from build123d import *

# Parameters (mm, degrees)
SKETCH3_W            = 36.5
SKETCH3_H            = 37.1
SHELL_DEPTH          = 8.6
SKETCH4_W            = 32.5
SKETCH4_H            = 31.1
MAIN_CAVITY_DEPTH    = 6.6
SKETCH5_W            = 32.5
SKETCH5_H            = 2
SUPPORT_SHELF_DEPTH  = 4.6
TERMINAL_INPUT_DEPTH = 2
SKETCH7_W            = 1.8
SKETCH7_H            = 3.6
MALE_TABS_DEPTH      = 2
SKETCH8_W            = 2
SKETCH8_H            = 4
FEMALE_TABS_DEPTH    = 2


with BuildPart() as part:
    # Sketch3 → Shell (new body)
    with BuildSketch(Plane(origin=(0, 0, 0), x_dir=(1, 0, 0), z_dir=(0, 1, 0))):
        with Locations((18.25, -18.55)):
            Rectangle(SKETCH3_W, SKETCH3_H)
    extrude(amount=SHELL_DEPTH)

    # Sketch4 → Main Cavity (cut)
    with BuildSketch(Plane(origin=(0, 8.6, 0), x_dir=(1, 0, 0), z_dir=(0, 1, 0))):
        with Locations((18.25, -19.55)):
            Rectangle(SKETCH4_W, SKETCH4_H)
    extrude(amount=-MAIN_CAVITY_DEPTH, mode=Mode.SUBTRACT)

    # Sketch5 → Support Shelf (cut)
    with BuildSketch(Plane(origin=(0, 8.6, 0), x_dir=(1, 0, 0), z_dir=(0, 1, 0))):
        with Locations((18.25, -3)):
            Rectangle(SKETCH5_W, SKETCH5_H)
    extrude(amount=-SUPPORT_SHELF_DEPTH, mode=Mode.SUBTRACT)

    # Sketch6 → Terminal Input (cut)
    with BuildSketch(Plane.XY.offset(37.1)):
        Polygon((31.2, 2.9), (31.2, 8.6), (4.1, 8.6), (4.1, 0), (14.7, 0), (14.7, 2.9), align=None)
    extrude(amount=-TERMINAL_INPUT_DEPTH, mode=Mode.SUBTRACT)

    # Sketch7 → Male Tabs (add)
    with BuildSketch(Plane(origin=(0, 8.6, 0), x_dir=(1, 0, 0), z_dir=(0, 1, 0))):
        with Locations((35.4, -27.1)):
            Rectangle(SKETCH7_W, SKETCH7_H)
        with Locations((0.9, -4.1)):
            Rectangle(SKETCH7_W, SKETCH7_H)
    extrude(amount=MALE_TABS_DEPTH)

    # Sketch8 → Female Tabs (cut)
    with BuildSketch(Plane(origin=(0, 8.6, 0), x_dir=(1, 0, 0), z_dir=(0, 1, 0))):
        with Locations((35.5, -4.3)):
            Rectangle(SKETCH8_W, SKETCH8_H)
        with Locations((1, -26.9)):
            Rectangle(SKETCH8_W, SKETCH8_H)
    extrude(amount=-FEMALE_TABS_DEPTH, mode=Mode.SUBTRACT)


solid = part.part
Can you work these out from the model? Positions are in its coordinate system, mm. A direction names the side the tool comes from. Round coordinates to 2 decimals unless told otherwise and drop trailing zeros. Loops run counter-clockwise (first coordinate to the right, second up) from the corner with the lowest first, then second, coordinate; pieces in that order, holes last. Notation, with made-up numbers: (10.25, 84.5) - (23.25, 84.5) arc R16 ccw to (23.25, 105.5) - close; hole circle Ø8 at (-12, -35.75). An arc over 180 degrees is marked (long way). Answer in a Markdown table with one row per item. Add a question column.
Q1. I want a section at A-A on x = 5. List the corners of the cut face in (y, z) for me, and give its area (3 significant figures).
Q2. I want a section at B-B on y = 9.25. List the corners of the cut face in (x, z) for me.
Q3. I want a section at D-D on y = 5.75. List the corners of the cut face in (x, z) for me.
Q4. For pin 1 Ø0.6 at (x, z) = (24.5, 2.5) entering from +Y; pin 2 Ø2 at (x, y) = (13, 3.5) entering from +Z; pin 3 Ø12 at (x, z) = (28, 31.5) entering from +Y, each with a flat end and sliding along its axis, tell me the tip position at first contact or that it passes through.
Q5. We'd pull the mould along Z, two halves only. Please class faces 1 (the flat face through (1, 8.6, 34)), 2 (the flat face through (2, 5, 19)), 3 (the flat face through (2, 4, 37.1)): pulls with the +Z half, pulls with the -Z half, needs draft (parallel to the pull), parting line crosses it, or undercut.
Q6. Which directions (+Z, -Z, +X, -X, +Y, -Y) give clear straight access to the entire face, cutting with the end or side of a thin tool? Please do faces 4 (the flat face through (1, 6.6, 27)), 5 (the flat face through (1, 10, 5.9)), 6 (the flat face through (31.2, 6, 36)).
Q7. I want a section at C-C on z = 8. List the corners of the cut face in (x, y) for me, and give its area (3 significant figures).
Q8. I need wall thicknesses on L1, parallel to X at y = 5.5, z = 16; L2, parallel to Z at x = 2.5, y = 7.25; L3, parallel to X at y = 1, z = 35.5. Which ranges of each line are inside material? Lowest first, please.
A:
| question | item | result |
|---|---|---|
| 1 | outline | (0, 0) - (8.6, 0) - (8.6, 2) - (4, 2) - (4, 4) - (2, 4) - (2, 35.1) - (0, 35.1) - close |
| 1 | area | 87.4 mm^2 |
| 2 | outline | (0, 2.3) - (1.8, 2.3) - (1.8, 5.9) - (0, 5.9) - close; (34.5, 25.3) - (36.3, 25.3) - (36.3, 28.9) - (34.5, 28.9) - close |
| 3 | outline | (0, 0) - (36.5, 0) - (36.5, 37.1) - (31.2, 37.1) - (31.2, 35.1) - (34.5, 35.1) - (34.5, 2) - (2, 2) - (2, 35.1) - (4.1, 35.1) - (4.1, 37.1) - (0, 37.1) - close |
| 4 | pin 1 | y = 4 |
| 4 | pin 2 | z = 4 |
| 4 | pin 3 | y = 8.6 |
| 5 | face 1 | needs draft |
| 5 | face 2 | undercut |
| 5 | face 3 | pulls with the +Z half |
| 6 | face 4 | -X, +Y |
| 6 | face 5 | +Z, +X, -X, +Y |
| 6 | face 6 | +Z, +Y |
| 7 | outline | (0, 0) - (36.5, 0) - (36.5, 8.6) - (34.5, 8.6) - (34.5, 2) - (2, 2) - (2, 8.6) - (0, 8.6) - close |
| 7 | area | 99.4 mm^2 |
| 8 | L1 | 0 to 2, 34.5 to 36.5 |
| 8 | L2 | 0 to 2, 35.1 to 37.1 |
| 8 | L3 | 0 to 4.1, 14.7 to 36.5 |
